Can you work these out from the model? Positions are in its coordinate system, mm. A direction names the side the tool comes from. Coordinates: 2 decimals unless noted, no trailing zeros. Write each loop counter-clockwise with the first axis right and the second up, starting at its lowest first coordinate (ties: lowest second). Pieces come first, ordered by that corner, then holes. Notation, with made-up numbers: (89, 50) - (139, 50) arc R23 cw to (139, 82) - close; hole circle Ø1 at (18, 31.25). An arc over 180 degrees is marked (long way). Use one line per item in the form item = value. Start each with the question number.
(1) For pin 1 Ø2 at (x, y) = (94.5, 3) entering from -Z; pin 2 Ø5 at (x, z) = (-121.5, 4) entering from -Y; pin 3 Ø1.5 at (x, z) = (43, 5.5) entering from +Y, each with a flat end and sliding along its axis, tell me the tip position at first contact or that it passes through.
(2) Thinking about a two-plate mould opening in X: for faces 1 (the face through (-126, 3, 5)), 2 (the face through (-119.6, 3.6, 2.6)), 3 (the face through (126, 3, 5)), 4 (the face through (-118, 6, 4)), which applies, pulls with the +X half, pulls with the -X half, needs draft (parallel to the pull), parting line crosses it, or undercut?
(3) On a 3-axis mill with a long thin cutter (end or side, diameter ignored), from which of +Z, -Z, +X, -X, +Y, -Y can I reach the whole of each face in a straight line? I mean faces 5 (the face through (122.4, 3.6, 2.6)), 6 (the face through (1.5, 2.5, 1.9)), 7 (the face through (116, 2, 0)). Say none if no direction works.
(4) If we section it at A-A on x = -84: Please give me the cut outline in (y, z), then the cut area to 3 significant figures.
(5) If I drill on probe 1 along X at (y, z) = (3.5, 4); probe 2 along X at (y, z) = (1.6, 4); probe 3 along Z at (x, y) = (-121, 4.8), over which ranges is the centre line in solid material (lowest first)? Write a range as from..to.
```python
from build123d import *

# Parameters (mm, degrees)
EXTRUDE_1_DEPTH             = 10
CUT_EXTRUDE_1_DEPTH         = 106
FILLET_1_R                  = 0.8
CUT_EXTRUDE_2_DEPTH         = 253.269696951
CHAMFER_1_SIZE              = 1
CHAMFER_1_SIZE2             = 1.137309439
SKETCH_7_W                  = 15
SKETCH_7_H                  = 2
CUT_EXTRUDE_3_DEPTH         = 1
HOLE_WIZARD_M21_D           = 1.6
HOLE_WIZARD_M21_DEPTH       = 6
HOLE_WIZARD_M21_CSINK_D     = 2.05
HOLE_WIZARD_M21_CSINK_ANGLE = 120
HOLE_WIZARD_M21_TIP         = 0.480688495
HOLE_WIZARD_M31_D           = 3.4
HOLE_WIZARD_M31_CBORE_D     = 6.5
HOLE_WIZARD_M31_CBORE_DEPTH = 3.6


with BuildPart() as part:
    # Эскиз1 → Бобышка-Вытянуть1 (new body)
    with BuildSketch(Plane.XY):
        Polygon((-126, 0), (126, 0), (126, 6), (111, 6), (111, 5), (-111, 5), (-111, 6), (-126, 6), align=None)
    extrude(amount=EXTRUDE_1_DEPTH)

    # Эскиз5 → Вырез-Вытянуть1 (cut, symmetric)
    with BuildSketch(Plane(origin=(0, 0, 0), x_dir=(0, 0, -1), z_dir=(1, 0, 0))):
        Polygon((0, 0), (-0.8, 0), (-3, 5), (0, 5), align=None)
    extrude(amount=CUT_EXTRUDE_1_DEPTH, both=True, mode=Mode.SUBTRACT)

    # Скругление1
    fillet_1_edges = [part.edges().sort_by_distance(p)[0] for p in [
        (-106, 2.5, 1.9),
        (106, 2.5, 1.9),
    ]]
    fillet(fillet_1_edges, radius=FILLET_1_R)

    # Эскиз6 → Вырез-Вытянуть2 (cut, through all)
    with BuildSketch(Plane.ZY.offset(126)):
        Polygon((1.3, 0), (10, 1), (10, 0), align=None)
    extrude(amount=-CUT_EXTRUDE_2_DEPTH, mode=Mode.SUBTRACT)

    # Фаска1
    chamfer_1_edges = [part.edges().sort_by_distance(p)[0] for p in [
        (0, 1, 10),
    ]]
    chamfer_1_side = [part.faces().sort_by_distance(p)[0] for p in [
        (0, 3.072254335, 10),
    ]]
    chamfer(chamfer_1_edges, length=CHAMFER_1_SIZE, length2=CHAMFER_1_SIZE2, reference=chamfer_1_side[0])

    # Эскиз7 → Вырез-Вытянуть3 (cut)
    with BuildSketch(Plane(origin=(0, 6, 0), x_dir=(1, 0, 0), z_dir=(0, 1, 0))):
        with Locations((-118.5, -9)):
            Rectangle(SKETCH_7_W, SKETCH_7_H)
        with Locations((118.5, -9)):
            Rectangle(SKETCH_7_W, SKETCH_7_H)
    extrude(amount=-CUT_EXTRUDE_3_DEPTH, mode=Mode.SUBTRACT)

    # Отверстие обработанное метчиком M21
    with Locations(Plane(origin=(0, 0, 0), x_dir=(-1, 0, 0), z_dir=(0, 0, -1))):
        with Locations((-116, 3.5), (116, 3.5)):
            CounterSinkHole(HOLE_WIZARD_M21_D / 2, HOLE_WIZARD_M21_CSINK_D / 2, depth=HOLE_WIZARD_M21_DEPTH, counter_sink_angle=HOLE_WIZARD_M21_CSINK_ANGLE)
            with Locations((0, 0, -(HOLE_WIZARD_M21_DEPTH + HOLE_WIZARD_M21_TIP / 2))):  # 118° drill point
                Cone(0, HOLE_WIZARD_M21_D / 2, HOLE_WIZARD_M21_TIP, mode=Mode.SUBTRACT)

    # Цековка для  винта с внутренним шестигранником M31 (through all)
    with Locations(Plane.XZ):
        with Locations((121, 4), (-121, 4)):
            CounterBoreHole(HOLE_WIZARD_M31_D / 2, HOLE_WIZARD_M31_CBORE_D / 2, HOLE_WIZARD_M31_CBORE_DEPTH)


solid = part.part
```
Reported:
q1.pin_1 = 1.68
q1.pin_2 = 3.6
q1.pin_3 = 5
q2.face_1 = pulls with the -X half
q2.face_2 = undercut
q2.face_3 = pulls with the +X half
q2.face_4 = needs draft
q3.face_5 = -Y
q3.face_6 = -Z, +Y
q3.face_7 = -Z, +X, -X, +Y, -Y
q4.outline = (0, 0.8) - (5, 3) - (5, 10) - (2, 10) - (0.87, 8.87) - (0, 1.3) - close
q4.area = 35.6 mm2
q5.probe_1 = -126..-124.25, -117.75..-116.8, -115.2..115.2, 116.8..117.75, 124.25..126
q5.probe_2 = -126..-124.25, -117.75..117.75, 124.25..126
q5.probe_3 = 0..2.3, 5.7..10
